Can you work these out from the drawing? Everything is in mm from the part's minimum corner. Coordinates: 2 decimals unless noted, no trailing zeros. Loops run counter-clockwise (first coordinate to the right, second up) from the corner with the lowest first, then second, coordinate; pieces in that order, holes last. Notation, with made-up numbers: M -16,47 L -7,47 A30 ccw -7,70 Z; hole C -37,-20 d11. An arc over 180 degrees is marked long. Write each question's results on one line, items separated by ' | '.
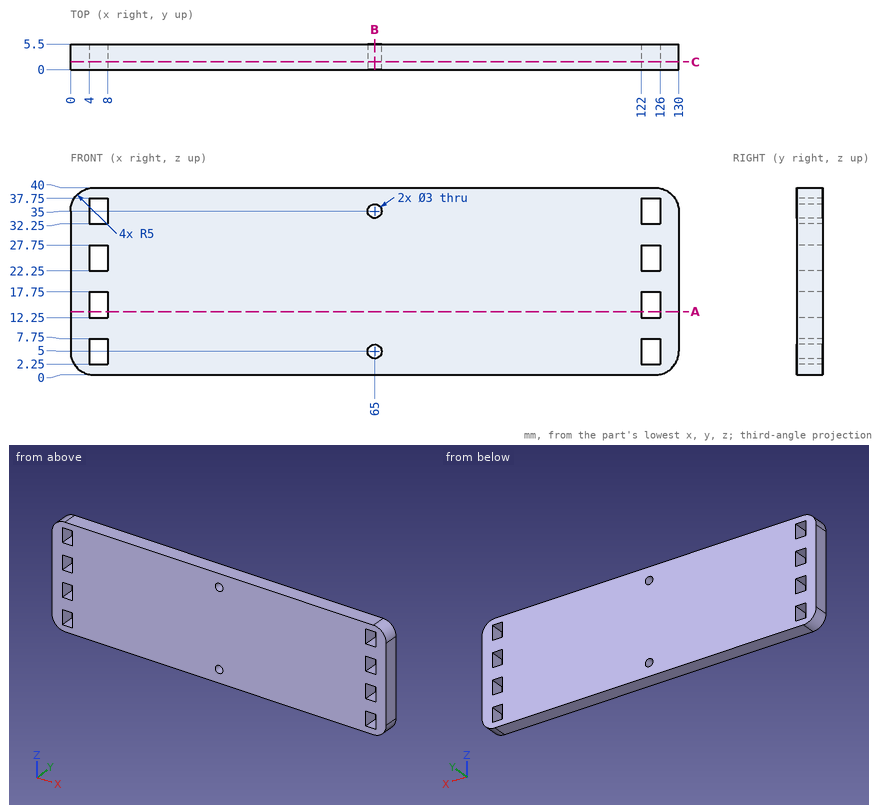
(1) Please list where these lines run through material, in increasing order: probe 1 along X at (y, z) = (2.3, 5); probe 2 along Z at (x, y) = (65, 3); probe 3 along X at (y, z) = (2.4, 7). Write a range as from..to.
Reported:
probe 1: x = 0..4, 8..63.5, 66.5..122, 126..130 | probe 2: z = 0..3.5, 6.5..33.5, 36.5..40 | probe 3: x = 0..4, 8..122, 126..130
(2) Imagine slicing it at C-C, the plane y = 1.7. State how many separate pieces and enclosed holes the cut face has, and give its area (3 significant figures).
Reported:
separate pieces: 1 | enclosed holes: 10 | area: 4,990 mm2
(3) Imagine slicing it at A-A, the plane z = 13.5. List the corners of the cut face in (x, y) for me, and give its area (3 significant figures).
Reported:
outline: M 0,0 L 4,0 L 4,5.5 L 0,5.5 Z; M 8,0 L 122,0 L 122,5.5 L 8,5.5 Z; M 126,0 L 130,0 L 130,5.5 L 126,5.5 Z | area: 671 mm2
(4) Imagine slicing it at B-B, the plane x = 65. List the corners of the cut face in (y, z) for me, and give its area (3 significant figures).
Reported:
outline: M 0,0 L 5.5,0 L 5.5,3.5 L 0,3.5 Z; M 0,6.5 L 5.5,6.5 L 5.5,33.5 L 0,33.5 Z; M 0,36.5 L 5.5,36.5 L 5.5,40 L 0,40 Z | area: 187 mm2
